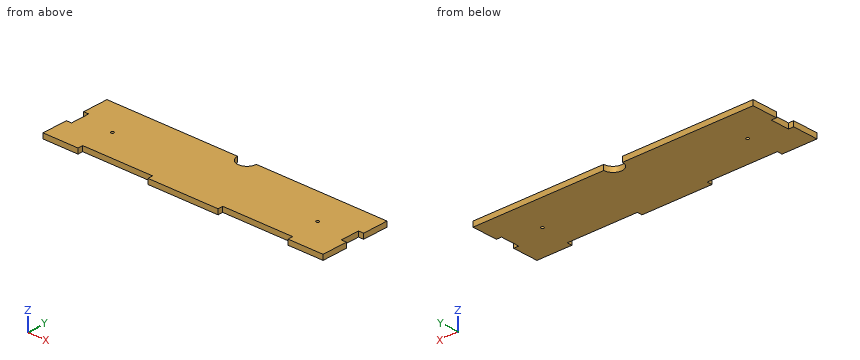
```python
from build123d import *

# Parameters (mm, degrees)
BOSS_EXTRUDE1_DEPTH = 5.5
SKETCH2_R           = 10
CUT_EXTRUDE2_DEPTH  = 311.022983019
SKETCH3_R           = 1.6
CUT_EXTRUDE3_DEPTH  = 311.022983019
SKETCH4_W           = 9.45
SKETCH4_H           = 3.25
SKETCH4_W_2         = 2.65
SKETCH4_H_2         = 1.25
SKETCH4_W_3         = 3.25
SKETCH4_H_3         = 9.45
SKETCH4_H_4         = 2.65
SKETCH4_W_4         = 1.25
BOSS_EXTRUDE2_DEPTH = 5.5


with BuildPart() as part:
    # Sketch1 → Boss-Extrude1 (new body)
    with BuildSketch(Plane.XY):
        Polygon((0, 78), (0, 50.625), (5.5, 50.625), (5.5, 42.125), (14.95, 42.125), (14.95, 43.375), (17.6, 43.375), (17.6, 42.125), (20.25, 42.125), (20.25, 38.875), (17.6, 38.875), (17.6, 37.625), (14.95, 37.625), (14.95, 38.875), (5.5, 38.875), (5.5, 30.375), (0, 30.375), (0, 3), (37.5, 3), (37.5, 8.5), (73.375, 8.5), (73.375, 17.95), (72.125, 17.95), (72.125, 20.6), (73.375, 20.6), (73.375, 23.25), (76.625, 23.25), (76.625, 20.6), (77.875, 20.6), (77.875, 17.95), (76.625, 17.95), (76.625, 8.5), (112.5, 8.5), (112.5, 3), (187.5, 3), (187.5, 8.5), (223.375, 8.5), (223.375, 17.95), (222.125, 17.95), (222.125, 20.6), (223.375, 20.6), (223.375, 23.25), (226.625, 23.25), (226.625, 20.6), (227.875, 20.6), (227.875, 17.95), (226.625, 17.95), (226.625, 8.5), (262.5, 8.5), (262.5, 3), (300, 3), (300, 30.375), (294.5, 30.375), (294.5, 38.875), (285.05, 38.875), (285.05, 37.625), (282.4, 37.625), (282.4, 38.875), (279.75, 38.875), (279.75, 42.125), (282.4, 42.125), (282.4, 43.375), (285.05, 43.375), (285.05, 42.125), (294.5, 42.125), (294.5, 50.625), (300, 50.625), (300, 78), align=None)
    extrude(amount=BOSS_EXTRUDE1_DEPTH)

    # Sketch2 → Cut-Extrude2 (cut, through all)
    with BuildSketch(Plane.XY):
        with Locations((150, 78)):
            Circle(SKETCH2_R)
    extrude(amount=CUT_EXTRUDE2_DEPTH, mode=Mode.SUBTRACT)

    # Sketch3 → Cut-Extrude3 (cut, through all)
    with BuildSketch(Plane.XY.offset(5.5)):
        with Locations((40, 40.5)):
            Circle(SKETCH3_R)
        with Locations((260, 40.5)):
            Circle(SKETCH3_R)
    extrude(amount=-CUT_EXTRUDE3_DEPTH, mode=Mode.SUBTRACT)

    # Sketch4 → Boss-Extrude2 (add)
    with BuildSketch(Plane.XY.offset(5.5)):
        with Locations((289.775, 40.5)):
            Rectangle(SKETCH4_W, SKETCH4_H)
        with Locations((283.725, 40.5)):
            Rectangle(SKETCH4_W_2, SKETCH4_H)
        with Locations((281.075, 40.5)):
            Rectangle(SKETCH4_W_2, SKETCH4_H)
        with Locations((283.725, 38.25)):
            Rectangle(SKETCH4_W_2, SKETCH4_H_2)
        with Locations((283.725, 42.75)):
            Rectangle(SKETCH4_W_2, SKETCH4_H_2)
        with Locations((225, 13.225)):
            Rectangle(SKETCH4_W_3, SKETCH4_H_3)
        with Locations((225, 19.275)):
            Rectangle(SKETCH4_W_3, SKETCH4_H_4)
        with Locations((225, 21.925)):
            Rectangle(SKETCH4_W_3, SKETCH4_H_4)
        with Locations((227.25, 19.275)):
            Rectangle(SKETCH4_W_4, SKETCH4_H_4)
        with Locations((222.75, 19.275)):
            Rectangle(SKETCH4_W_4, SKETCH4_H_4)
        with Locations((75, 13.225)):
            Rectangle(SKETCH4_W_3, SKETCH4_H_3)
        with Locations((75, 19.275)):
            Rectangle(SKETCH4_W_3, SKETCH4_H_4)
        with Locations((75, 21.925)):
            Rectangle(SKETCH4_W_3, SKETCH4_H_4)
        with Locations((77.25, 19.275)):
            Rectangle(SKETCH4_W_4, SKETCH4_H_4)
        with Locations((72.75, 19.275)):
            Rectangle(SKETCH4_W_4, SKETCH4_H_4)
        with Locations((10.225, 40.5)):
            Rectangle(SKETCH4_W, SKETCH4_H)
        with Locations((16.275, 40.5)):
            Rectangle(SKETCH4_W_2, SKETCH4_H)
        with Locations((16.275, 38.25)):
            Rectangle(SKETCH4_W_2, SKETCH4_H_2)
        with Locations((18.925, 40.5)):
            Rectangle(SKETCH4_W_2, SKETCH4_H)
        with Locations((16.275, 42.75)):
            Rectangle(SKETCH4_W_2, SKETCH4_H_2)
    extrude(amount=-BOSS_EXTRUDE2_DEPTH)


solid = part.part
```
Geometry check sheet. Reference: the model listing, model coordinates, mm. Round coordinates to 2 decimals unless told otherwise and drop trailing zeros. Order: outer loops, then holes, each group sorted by start corner. A loop starts at its lowest first (then second) coordinate and runs counter-clockwise, first axis right, second up. Notation, with made-up numbers: (-9.5, 24) - (-1.5, 24) arc R19 ccw to (-1.5, 61) - close; hole circle Ø8 at (61, 8.5). An arc over 180 degrees is marked (long way). Use a Markdown table: item, result. Add a question column.
(1) Material ranges on line 1 along Y through (x, z) = (260, 4.05); line 2 along Y through (x, z) = (83.5, 5.2); line 3 along X through (y, z) = (33.5, 4.55), recorded low to high. Write a range as [from, to].
(2) Sectioned sample at D-D, the plane y = 47. Enter the section's corners in (x, z).
(3) Sectioned sample at B-B, the plane y = 73.5. Enter the section's corners in (x, z).
(4) Sectioned sample at C-C, the plane x = 83. Enter the section's corners in (y, z).
(5) Depth check by flat-ended pin: pin 1 (1.6 mm diameter, centred on x = 214, z = 3, fed in from -Y); pin 2 (2.5 mm diameter, centred on x = 260, y = 40.5, fed in from -Z); pin 3 (3 mm diameter, centred on y = 42, z = 3, fed in from +X); pin 4 (3 mm diameter, centred on y = 36.5, z = 1.5, fed in from -X). Enter the tip coordinate at first touch or a pass-through.
(6) Sectioned sample at A-A, the plane z = 1.5. Enter the section's corners in (x, y) (3 decimals), and give its area (3 significant figures).
Answers below:
| question | item | result |
|---|---|---|
| 1 | line 1 | [8.5, 38.9], [42.1, 78] |
| 1 | line 2 | [8.5, 78] |
| 1 | line 3 | [5.5, 294.5] |
| 2 | outline | (5.5, 0) - (294.5, 0) - (294.5, 5.5) - (5.5, 5.5) - close |
| 3 | outline | (0, 0) - (141.07, 0) - (141.07, 5.5) - (0, 5.5) - close; (158.93, 0) - (300, 0) - (300, 5.5) - (158.93, 5.5) - close |
| 4 | outline | (8.5, 0) - (78, 0) - (78, 5.5) - (8.5, 5.5) - close |
| 5 | pin 1 | y = 8.5 |
| 5 | pin 2 | through |
| 5 | pin 3 | x = 294.5 |
| 5 | pin 4 | x = 5.5 |
| 6 | outline | (0, 3) - (37.5, 3) - (37.5, 8.5) - (112.5, 8.5) - (112.5, 3) - (187.5, 3) - (187.5, 8.5) - (262.5, 8.5) - (262.5, 3) - (300, 3) - (300, 30.375) - (294.5, 30.375) - (294.5, 50.625) - (300, 50.625) - (300, 78) - (160, 78) arc R10 cw to (140, 78) - (0, 78) - (0, 50.625) - (5.5, 50.625) - (5.5, 30.375) - (0, 30.375) - close; hole circle Ø3.2 at (40, 40.5); hole circle Ø3.2 at (260, 40.5) |
| 6 | area | 21,300 mm² |
